from build123d import *

# Parameters (mm, degrees)
BOSS_EXTRUDE1_DEPTH      = 0.1
BOSS_EXTRUDE1_DEPTH_BACK = 0.6
BOSS_EXTRUDE2_DEPTH      = 0.3
SKETCH3_W                = 0.8
SKETCH3_H                = 2.9
SKETCH3_H_2              = 3.2
BOSS_EXTRUDE3_DEPTH      = 0.05
CUT_EXTRUDE1_DEPTH       = 0.7
FILLET1_R                = 0.5
FILLET2_R                = 0.08


with BuildPart() as part:
    # Sketch1 → Boss-Extrude1 (new body, two sides)
    with BuildSketch(Plane.XY) as boss_extrude1_sk:
        Polygon((-5.5, 30.230563632), (5.5, 30.230563632), (5.5, 21.530563632), (4.2, 20.230563632), (4.2, 15.230563632), (-5.5, 15.230563632), align=None)
    extrude(amount=BOSS_EXTRUDE1_DEPTH)
    extrude(boss_extrude1_sk.sketch, amount=-BOSS_EXTRUDE1_DEPTH_BACK)

    # Sketch2 → Boss-Extrude2 (add)
    with BuildSketch(Plane(origin=(0, 0, -0.6), x_dir=(-1, 0, 0), z_dir=(0, 0, -1))):
        with BuildLine():
            Line((-5.5, 30.230563632), (5.5, 30.230563632))
            Line((5.5, 30.230563632), (5.5, 29.030563632))
            ThreePointArc((5.5, 29.030563632), (0, 28.430563632), (-5.5, 29.030563632))
            Line((-5.5, 29.030563632), (-5.5, 30.230563632))
        make_face()
    extrude(amount=BOSS_EXTRUDE2_DEPTH)

    # Sketch3 → Boss-Extrude3 (add)
    with BuildSketch(Plane.XY.offset(0.1)):
        with Locations((-4.5, 17.780563632)):
            Rectangle(SKETCH3_W, SKETCH3_H)
        with Locations((3.2, 17.780563632)):
            Rectangle(SKETCH3_W, SKETCH3_H)
        with Locations((-3.4, 17.780563632)):
            Rectangle(SKETCH3_W, SKETCH3_H)
        with Locations((-1.2, 17.780563632)):
            Rectangle(SKETCH3_W, SKETCH3_H)
        with Locations((1, 17.780563632)):
            Rectangle(SKETCH3_W, SKETCH3_H)
        with Locations((2.1, 17.780563632)):
            Rectangle(SKETCH3_W, SKETCH3_H)
        with Locations((-2.3, 17.630563632)):
            Rectangle(SKETCH3_W, SKETCH3_H_2)
        with Locations((-0.1, 17.630563632)):
            Rectangle(SKETCH3_W, SKETCH3_H_2)
    extrude(amount=BOSS_EXTRUDE3_DEPTH)

    # Sketch4 → Cut-Extrude1 (cut)
    with BuildSketch(Plane(origin=(0, 0, -0.6), x_dir=(-1, 0, 0), z_dir=(0, 0, -1))):
        Polygon((-5.5, 23.130563632), (-5.5, 25.030563632), (-4.8, 24.330563632), (-4.8, 23.130563632), align=None)
    extrude(amount=-CUT_EXTRUDE1_DEPTH, mode=Mode.SUBTRACT)

    # Fillet1
    fillet1_edges = [part.edges().sort_by_distance(p)[0] for p in [
        (-5.5, 15.230563632, -0.25),
        (-5.5, 30.230563632, -0.4),
        (5.5, 30.230563632, -0.4),
        (4.2, 15.230563632, -0.25),
    ]]
    fillet(fillet1_edges, radius=FILLET1_R)

    # Fillet2
    fillet2_edges = [part.edges().sort_by_distance(p)[0] for p in [
        (4.85, 20.880563632, 0.1),
        (5.5, 21.530563632, -0.25),
        (4.2, 20.230563632, -0.25),
        (5.5, 22.330563632, 0.1),
        (5.5, 22.330563632, -0.6),
        (4.85, 20.880563632, -0.6),
        (5.5, 27.030563632, -0.6),
        (5.5, 27.380563632, 0.1),
        (5.5, 25.030563632, -0.25),
        (4.8, 24.330563632, -0.25),
        (4.8, 23.130563632, -0.25),
        (5.5, 23.130563632, -0.25),
        (5.15, 24.680563632, -0.6),
        (5.15, 23.130563632, -0.6),
        (4.8, 23.730563632, -0.6),
        (5.15, 24.680563632, 0.1),
        (4.8, 23.730563632, 0.1),
        (5.15, 23.130563632, 0.1),
        (0, 30.230563632, -0.9),
        (0, 30.230563632, 0.1),
        (5.5, 29.380563632, -0.9),
        (-5.353553391, 30.084117023, -0.9),
        (5.353553391, 30.084117023, -0.9),
        (-5.5, 22.730563632, 0.1),
        (-0.65, 15.230563632, 0.1),
        (4.2, 17.980563632, 0.1),
        (4.053553391, 15.377010242, 0.1),
        (-5.353553391, 15.377010242, 0.1),
        (-5.353553391, 30.084117023, 0.1),
        (5.353553391, 30.084117023, 0.1),
        (-0.65, 15.230563632, -0.6),
        (4.2, 17.980563632, -0.6),
        (4.053553391, 15.377010242, -0.6),
        (-5.353553391, 15.377010242, -0.6),
        (-5.5, 22.380563632, -0.6),
        (0, 28.430563632, -0.6),
        (5.5, 29.030563632, -0.75),
        (-5.5, 29.030563632, -0.75),
        (0, 28.430563632, -0.9),
        (-5.5, 29.380563632, -0.9),
    ]]
    fillet(fillet2_edges, radius=FILLET2_R)


solid = part.part
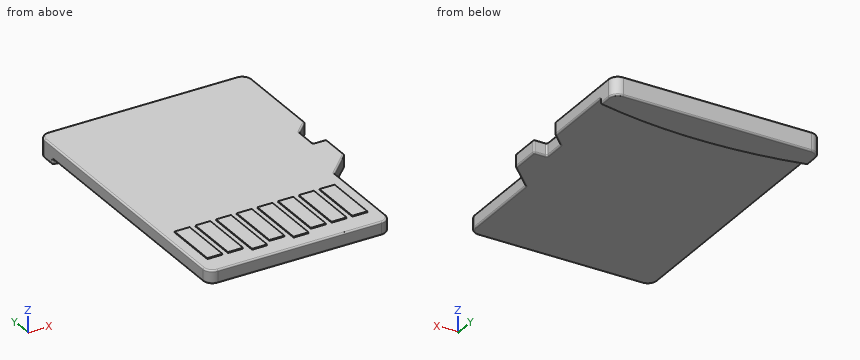
Source: CAD feature listing. Evaluate the final solid. Frame: model axes, mm. Round coordinates to 2 decimals unless told otherwise and drop trailing zeros. Loops run counter-clockwise (first coordinate to the right, second up) from the corner with the lowest first, then second, coordinate; pieces in that order, holes last. Notation, with made-up numbers: (-5, 80.25) - (45, 80.25) arc R18 ccw to (45, 104.25) - close; hole circle Ø1 at (-31.75, 6). An arc over 180 degrees is marked (long way). Write item = value, one per line. Start each with the question number.
Item 1: Section query A-A on z = -0.3. Output: boundary loops of the cut face in (x, y).
Item 2: Material intervals for line 1 (Z direction, x = 2, y = 28); line 2 (Z direction, x = 1.5, y = 29); line 3 (X direction, y = 23.75, z = -0.5), sorted ascending.
Item 3: Section query B-B on y = 19.75. Output: boundary loops of the cut face in (x, z), plus the area to 3 significant figures.
Item 4: First-contact query: pin 1 Ø2 at (x, y) = (0, 24) entering from -Z; pin 2 Ø4 at (x, y) = (-4.5, 26) entering from +Z. Flat tips, straight axial feed; report the tip coordinate or a pass-through.
Results list:
q1.outline = (-5.5, 15.73) arc R0.5 ccw to (-5, 15.23) - (3.7, 15.23) arc R0.5 ccw to (4.2, 15.73) - (4.2, 20.2) arc R0.08 cw to (4.22, 20.25) - (5.48, 21.51) arc R0.08 ccw to (5.5, 21.56) - (5.5, 23.05) arc R0.08 ccw to (5.42, 23.13) - (4.88, 23.13) arc R0.08 cw to (4.8, 23.21) - (4.8, 24.3) arc R0.08 cw to (4.82, 24.35) - (5.48, 25.01) arc R0.08 ccw to (5.5, 25.06) - (5.5, 29.73) arc R0.5 ccw to (5, 30.23) - (-5, 30.23) arc R0.5 ccw to (-5.5, 29.73) - close
q2.line_1 = -0.6 to 0.1
q2.line_2 = -0.9 to 0.1
q2.line_3 = -5.5 to 4.8
q3.outline = (-5.5, -0.52) arc R0.08 ccw to (-5.42, -0.6) - (4.12, -0.6) arc R0.08 ccw to (4.2, -0.52) - (4.2, 0.02) arc R0.08 ccw to (4.12, 0.1) - (-5.42, 0.1) arc R0.08 ccw to (-5.5, 0.02) - close
q3.area = 6.78 mm²
q4.pin_1 = -0.6
q4.pin_2 = 0.1
